For this review, take the finished solid that the model builds, in its own axes (mm). Face numbers are marked on the shaded views. Round coordinates to 2 decimals unless told otherwise and drop trailing zeros. Order: outer loops, then holes, each group sorted by start corner. A loop starts at its lowest first (then second) coordinate and runs counter-clockwise, first axis right, second up.
```python
from build123d import *

# Parameters (mm, degrees)
SKETCH_1_W          = 8
SKETCH_1_H          = 8
EXTRUDE_1_DEPTH     = 34
SKETCH_2_R          = 1.7
CUT_EXTRUDE_1_DEPTH = 34
SKETCH_3_R          = 1.7
CUT_EXTRUDE_2_DEPTH = 34


with BuildPart() as part:
    # 草图1 → 凸台-拉伸1 (new body)
    with BuildSketch(Plane(origin=(0, 0, 0), x_dir=(1, 0, 0), z_dir=(0, 1, 0))):
        Rectangle(SKETCH_1_W, SKETCH_1_H)
    extrude(amount=EXTRUDE_1_DEPTH)

    # 草图2 → 切除-拉伸1 (cut)
    with BuildSketch(Plane(origin=(0, 0, -4), x_dir=(-1, 0, 0), z_dir=(0, 0, -1))):
        with Locations((0, 29)):
            Circle(SKETCH_2_R)
        with Locations((0, 13)):
            Circle(SKETCH_2_R)
    extrude(amount=-CUT_EXTRUDE_1_DEPTH, mode=Mode.SUBTRACT)

    # 草图3 → 切除-拉伸2 (cut)
    with BuildSketch(Plane(origin=(4, 0, 0), x_dir=(0, 0, -1), z_dir=(1, 0, 0))):
        with Locations((0, 5)):
            Circle(SKETCH_3_R)
        with Locations((0, 21)):
            Circle(SKETCH_3_R)
    extrude(amount=-CUT_EXTRUDE_2_DEPTH, mode=Mode.SUBTRACT)


solid = part.part
```
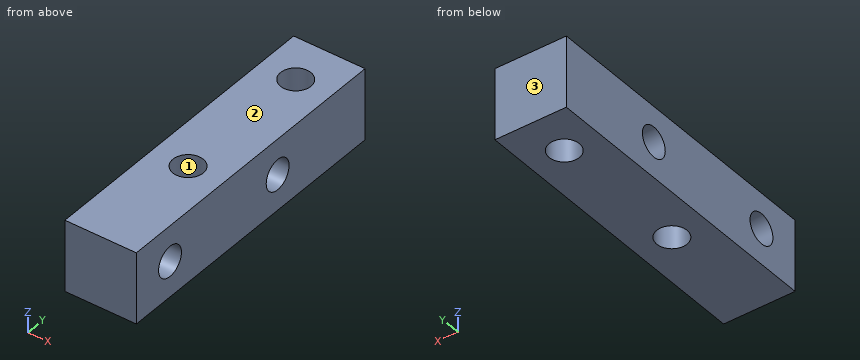
Q1. Take a section at A-A, the plane z = 0. State the section outline as (x, y) points, plus the area to 3 significant figures.
Q2. Take a section at D-D, the plane z = 2.5. State the section outline as (x, y) points.
Q3. Clearance check with a flat-ended pin moving along its axis: pin 1 (2.5 mm diameter, centred on y = 5, z = 0, fed in from +X). State where the tip first meets the part, or that it passes through.
Q4. Wall thickness on line 1 (Y direction, x = 0, z = 2); line 2 (Y direction, x = -1.5, z = -1.5); line 3 (Y direction, x = 1.5, z = -3.5): over which ranges is each line inside the solid? List them lowest first.
Q5. Take a section at C-C, the plane y = 29. State the section outline as (x, z) points.
Q6. Take a section at B-B, the plane x = 0. State the section outline as (y, z) points.
Q7. Mouldability with a two-part tool opening along Y and no side actions: class the marked faces 1, 2 and 3 as +Y half, -Y half, draft (parallel to the pull), parting line (faces both ways), or undercut.
Working result:
1. outline: (-4, 0) - (4, 0) - (4, 3.3) - (-4, 3.3) - close; (-4, 6.7) - (4, 6.7) - (4, 19.3) - (-4, 19.3) - close; (-4, 22.7) - (4, 22.7) - (4, 34) - (-4, 34) - close; hole circle Ø3.4 at (0, 13); hole circle Ø3.4 at (0, 29)
1. area: 199 mm2
2. outline: (-4, 0) - (4, 0) - (4, 34) - (-4, 34) - close; hole circle Ø3.4 at (0, 13); hole circle Ø3.4 at (0, 29)
3. pin 1: passes through
4. line 1: y = 0 to 11.3, 14.7 to 27.3, 30.7 to 34
4. line 2: y = 0 to 4.2, 5.8 to 12.2, 13.8 to 20.2, 21.8 to 28.2, 29.8 to 34
4. line 3: y = 0 to 12.2, 13.8 to 28.2, 29.8 to 34
5. outline: (-4, -4) - (-1.7, -4) - (-1.7, 4) - (-4, 4) - close; (1.7, -4) - (4, -4) - (4, 4) - (1.7, 4) - close
6. outline: (0, -4) - (11.3, -4) - (11.3, 4) - (0, 4) - close; (14.7, -4) - (27.3, -4) - (27.3, 4) - (14.7, 4) - close; (30.7, -4) - (34, -4) - (34, 4) - (30.7, 4) - close; hole circle Ø3.4 at (5, 0); hole circle Ø3.4 at (21, 0)
7. face 1: undercut
7. face 2: draft
7. face 3: +Y half
